Model file for the job. Use its own axes, mm. Face numbers are marked on the shaded views. A direction names the side the tool comes from. Coordinates: 2 decimals unless noted, no trailing zeros. Loops run counter-clockwise (first coordinate to the right, second up) from the corner with the lowest first, then second, coordinate; pieces in that order, holes last.
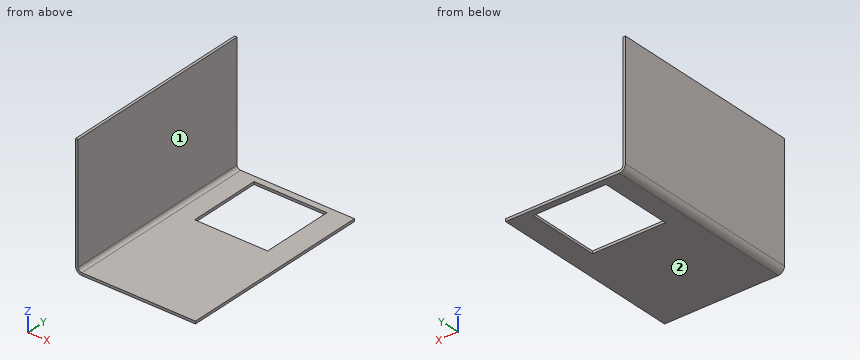
Autodesk Inventor part; units mm, degrees
ref_plane "YZ Plane" through (0, 0, 0) normal (1, 0, 0) x (0, 1, 0)
ref_plane "XZ Plane" through (0, 0, 0) normal (0, 1, 0) x (-1, 0, 0)
ref_plane "XY Plane" through (0, 0, 0) normal (0, 0, 1) x (1, 0, 0)
sketch "Sketch1" plane through (0, 0, 0) normal (0, 0, 1) x (1, 0, 0)
  line L0 (-46, -75) -> (46, -75)
  line L1 (46, -75) -> (46, 75)
  line L2 (46, 75) -> (-46, 75)
  line L3 (-46, 75) -> (-46, -75)
  line L4 (-46, -75) -> (46, 75) construction
  line L5 (46, -75) -> (-46, 75) construction
  point P0 (0, 0)
  dimension "d154" = 92
  dimension "d155" = 150
extrude "Plate5" add sketch "Sketch1" along normal blind 2
sketch "Sketch7" plane through (-44, -75, 0) normal (-1, 0, 0) x (0, -1, 0)
  line L0 (-150, 0) -> (0, 0)
  line L1 (0, 0) -> (0, 94)
  line L2 (0, 94) -> (-150, 94)
  line L3 (-150, 94) -> (-150, 0)
edge flange "Flange3" height 94 angle 90 thickness 2 bend radius 2.75 thickness toward (-1, 0, 0) relief round relief width 2 relief depth 1 edges at (-46, 0, 2) wall of the first edge with corners at (-44, 75, 0) (-44, -75, 0) (-44, -75, 94) (-44, 75, 94)
bend "Bend3"
corner "Corner3"
sketch "Sketch8" plane through (0, 0, 2) normal (0, 0, 1) x (1, 0, 0)
  line L0 (46, 75) -> (46, -75)
  line L1 (-41.25, 75) -> (46, 75)
  line L2 (29, 70) -> (-27, 70)
  line L3 (-27, 70) -> (-27, 14)
  line L4 (-27, 14) -> (29, 14)
  line L5 (29, 14) -> (29, 70)
  line L6 (29, 70) -> (-27, 14) construction
  line L7 (-27, 70) -> (29, 14) construction
  point P0 (0, 0)
  point P1 (1, 42)
  point P2 (2.375, 75)
  dimension "d167" = 56
  dimension "d168" = 56
  dimension "d169" = 5
  dimension "d172" = 17
extrude "Cut1" cut sketch "Sketch8" against normal blind 2
properties part number "APN 752 FDS 1200 FLANGE 2" material "Stainless Steel"
Q1. Drill centre lines: line 1 (Z direction, x = 26.5, y = -59); line 2 (X direction, y = 56.5, z = 75). Where is each one in solid material? Low to high.
Answers:
line 1: z = 0 to 2
line 2: x = -46 to -44
Q2. Slice it at C-C (y = -12). List the corners of the cut face in (x, z), and give its area (3 significant figures).
Answers:
outline: (-46, 4.75) arc R4.75 ccw to (-41.25, 0) - (46, 0) - (46, 2) - (-41.25, 2) arc R2.75 cw to (-44, 4.75) - (-44, 94) - (-46, 94) - close
area: 365 mm2
Q3. Flat gauge pins, fed straight in: P1, Ø2, axis at y = 53, z = 0.5, coming from the -X side; P2, Ø3, axis at x = -29.5, y = -2.5, coming from the +Z side; P3, Ø10, axis at y = 35.5, z = 55, coming from the +X side. Where does each tip first touch, or does it go through?
Answers:
P1: stops at x = -44.71
P2: stops at z = 2
P3: stops at x = -44
Q4. Slice it at B-B (y = 28.5). List the corners of the cut face in (x, z), and give its area (3 significant figures).
Answers:
outline: (-46, 4.75) arc R4.75 ccw to (-41.25, 0) - (-27, 0) - (-27, 2) - (-41.25, 2) arc R2.75 cw to (-44, 4.75) - (-44, 94) - (-46, 94) - close; (29, 0) - (46, 0) - (46, 2) - (29, 2) - close
area: 253 mm2
Q5. Slice it at D-D (z = 56). List the corners of the cut face in (x, y).
Answers:
outline: (-46, -75) - (-44, -75) - (-44, 75) - (-46, 75) - close
Q6. Slice it at A-A (x = -12.5). List the corners of the cut face in (y, z).
Answers:
outline: (-75, 0) - (14, 0) - (14, 2) - (-75, 2) - close; (70, 0) - (75, 0) - (75, 2) - (70, 2) - close
Q7. Which spindle directions (+Z, -Z, +X, -X, +Y, -Y) get a long thin tool onto all of the face, cutting with end or side? Do the marked faces 1 and 2. Say none if no direction does.
Answers:
face 1: +Z, +X, +Y, -Y
face 2: -Z, +X, -X, +Y, -Y
